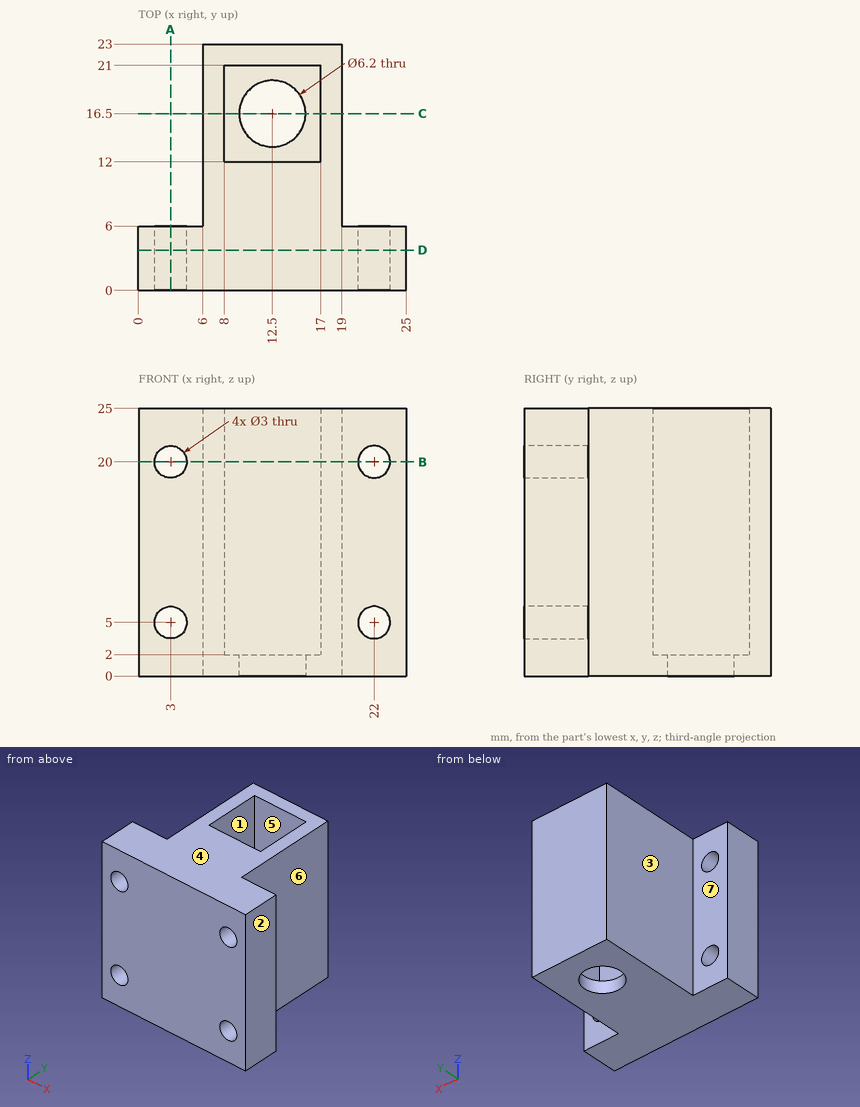
For this review, use the dimensioned drawing (mm, ordinates from the lowest corner) and the shaded views. A direction names the side the tool comes from. Round coordinates to 2 decimals unless told otherwise and drop trailing zeros. Order: outer loops, then holes, each group sorted by start corner. A loop starts at its lowest first (then second) coordinate and runs counter-clockwise, first axis right, second up. Notation, with made-up numbers: M 36.5,-31.5 L 95.5,-31.5 A10 ccw 95.5,-20.5 Z; hole C -10,-23 d3. An arc over 180 degrees is marked long. Use a Markdown table: item, result. Add a question column.
Item 1: Tool access review of the marked faces 5, 6 and 7: name each direction out of +Z, -Z, +X, -X, +Y, -Y from which nothing blocks a thin tool from reaching the whole face with its end or side.
Item 2: Insertion check: pin 1 (2 mm diameter, centred on y = 15.5, z = 16.5, fed in from +X); pin 2 (6 mm diameter, centred on x = 12.5, y = 13, fed in from +Z); pin 3 (13.5 mm diameter, centred on y = 16, z = 18, fed in from -X); pin 4 (6.5 mm diameter, centred on x = 23, z = 10.5, fed in from +Y). Each pin has a flat end and moves straight along its axis. Give the tip position at first contact, or say it passes through.
Item 3: Mouldability with a two-part tool opening along X and no side actions: class the marked faces 1, 2, 3 and 4 as released by +X, released by -X, zero draft, split by the parting line, or undercut.
Item 4: To check wall thickness, follow line 1 along Z through (x, y) = (22, 2.45); line 2 along Y through (x, z) = (9.5, 9); line 3 along X through (y, z) = (15, 22.75). State the ranges of each line that lie inside material, in increasing order.
Item 5: Add section C-C, the plane y = 16.5. Give the boundary of the cut face in (x, z), then the cut area to 3 significant figures.
Item 6: Add section D-D, the plane y = 3.75. Give the boundary of the cut face in (x, z), then the cut area to 3 significant figures.
Item 7: Add section A-A, the plane x = 3. Give the boundary of the cut face in (y, z).
Item 8: Add section B-B, the plane z = 20. Give the boundary of the cut face in (x, y).
Geometry results:
| question | item | result |
|---|---|---|
| 1 | face 5 | +Z |
| 1 | face 6 | +Z, -Z, +X, +Y |
| 1 | face 7 | +Z, -Z, -X, +Y |
| 2 | pin 1 | stops at x = 19 |
| 2 | pin 2 | stops at z = 25 |
| 2 | pin 3 | stops at x = 6 |
| 2 | pin 4 | stops at y = 6 |
| 3 | face 1 | undercut |
| 3 | face 2 | released by +X |
| 3 | face 3 | released by -X |
| 3 | face 4 | zero draft |
| 4 | line 1 | z = 0 to 3.5, 6.5 to 18.5, 21.5 to 25 |
| 4 | line 2 | y = 0 to 12, 21 to 23 |
| 4 | line 3 | x = 6 to 8, 17 to 19 |
| 5 | outline | M 6,0 L 9.4,0 L 9.4,2 L 8,2 L 8,25 L 6,25 Z; M 15.6,0 L 19,0 L 19,25 L 17,25 L 17,2 L 15.6,2 Z |
| 5 | area | 106 mm² |
| 6 | outline | M 0,0 L 25,0 L 25,25 L 0,25 Z; hole C 3,5 d3; hole C 3,20 d3; hole C 22,5 d3; hole C 22,20 d3 |
| 6 | area | 597 mm² |
| 7 | outline | M 0,0 L 6,0 L 6,3.5 L 0,3.5 Z; M 0,6.5 L 6,6.5 L 6,18.5 L 0,18.5 Z; M 0,21.5 L 6,21.5 L 6,25 L 0,25 Z |
| 8 | outline | M 0,0 L 1.5,0 L 1.5,6 L 0,6 Z; M 4.5,0 L 20.5,0 L 20.5,6 L 19,6 L 19,23 L 6,23 L 6,6 L 4.5,6 Z; M 23.5,0 L 25,0 L 25,6 L 23.5,6 Z; hole M 8,12 L 17,12 L 17,21 L 8,21 Z |
